Could you check a few things on this model? Use its own coordinates, in mm. Round coordinates to 2 decimals unless told otherwise and drop trailing zeros. Write each loop counter-clockwise with the first axis right and the second up, starting at its lowest first coordinate (ties: lowest second). Pieces come first, ordered by that corner, then holes. Notation, with made-up numbers: (31, 63.5) -> (78, 63.5) arc R22 cw to (78, 72.5) -> close; hole circle Ø2 at (4, 1). An arc over 180 degrees is marked (long way). Answer in a Markdown table with one row per item.
Autodesk Inventor part; units mm, degrees
ref_plane "YZ Plane" through (0, 0, 0) normal (1, 0, 0) x (0, 1, 0)
ref_plane "XZ Plane" through (0, 0, 0) normal (0, 1, 0) x (-1, 0, 0)
ref_plane "XY Plane" through (0, 0, 0) normal (0, 0, 1) x (1, 0, 0)
sketch "Sketch1" plane through (0, 0, 0) normal (0, 1, 0) x (-1, 0, 0)
  line L0 (945.4953, -52.3895) -> (1058.1259, -52.3895)
  arc A0 (945.4953, 55.8486) -> (981.8106, 103.6105) centre (854.964, 162.3701) ccw
  arc A1 (1021.8106, 103.6105) -> (1058.1259, 55.8486) centre (1148.6572, 162.3701) ccw
  line L1 (967.8106, 44.6105) -> (967.8106, 29.6105)
  line L2 (967.8106, -8.3895) -> (967.8106, -23.3895)
  line L3 (967.8106, 44.6105) -> (964.8106, 44.6105)
  line L4 (964.8106, 44.6105) -> (964.8106, 29.6105)
  line L5 (964.8106, 29.6105) -> (967.8106, 29.6105)
  line L6 (967.8106, -23.3895) -> (964.8106, -23.3895)
  line L7 (964.8106, -23.3895) -> (964.8106, -8.3895)
  line L8 (964.8106, -8.3895) -> (967.8106, -8.3895)
  line L9 (1035.8106, 44.6105) -> (1035.8106, 29.6105)
  line L10 (1035.8106, -8.3895) -> (1035.8106, -23.3895)
  line L11 (1035.8106, 44.6105) -> (1038.8106, 44.6105)
  line L12 (1038.8106, 44.6105) -> (1038.8106, 29.6105)
  line L13 (1038.8106, 29.6105) -> (1035.8106, 29.6105)
  line L14 (1035.8106, -23.3895) -> (1038.8106, -23.3895)
  line L15 (1038.8106, -23.3895) -> (1038.8106, -8.3895)
  line L16 (1038.8106, -8.3895) -> (1035.8106, -8.3895)
  line L17 (1058.1259, 55.8486) -> (1058.1259, -52.3895)
  line L18 (945.4953, 55.8486) -> (945.4953, -52.3895)
  line L19 (1001.8106, 123.6105) -> (1003.3106, 123.6105)
  line L20 (1003.3106, 123.6105) -> (1003.3106, 115.6105)
  line L21 (1003.3106, 111.6105) -> (1000.3106, 111.6105)
  line L22 (1000.3106, 115.6105) -> (1000.3106, 123.6257)
  line L23 (1000.3106, 123.6257) -> (1001.8106, 123.6105)
  line L24 (1003.3106, 115.6105) -> (1003.3106, 111.6105)
  line L25 (1000.3106, 115.6105) -> (1000.3106, 111.6105)
  arc A2 (1012.3106, 159.6326) -> (991.3106, 159.6326) centre (1001.8106, 142.6105) ccw
  arc A3 (981.8106, 103.6105) -> (991.3106, 159.6326) centre (700.3575, 180.1548) ccw
  arc A4 (1012.3106, 159.6326) -> (1021.8106, 103.6105) centre (1303.2637, 180.1548) ccw
  arc A5 (945.4953, 55.8486) -> (981.8106, 103.6105) centre (854.964, 162.3701) ccw
  arc A6 (1021.8106, 103.6105) -> (1058.1259, 55.8486) centre (1148.6572, 162.3701) ccw
  line L26 (1001.8106, 123.6105) -> (1003.3106, 123.6105)
  line L27 (1003.3106, 123.6105) -> (1003.3106, 115.6105)
  line L28 (1003.3106, 111.6105) -> (1000.3106, 111.6105)
  line L29 (1000.3106, 115.6105) -> (1000.3106, 123.6105)
  line L30 (1000.3106, 123.6105) -> (1001.8106, 123.6105)
  line L31 (1000.3106, 111.6105) -> (1000.3106, 115.6105)
  line L32 (1003.3106, 111.6105) -> (1003.3106, 115.6105)
  line L33 (1001.8106, 103.6105) -> (1086.8106, 103.6105) construction
  line L34 (1001.8106, 103.6105) -> (916.8106, 103.6105) construction
  line L35 (1086.8106, 133.6105) -> (1071.8106, 133.6105) construction
  line L36 (1071.8106, 133.6105) -> (1071.8106, 73.6105) construction
  line L37 (1071.8106, 73.6105) -> (1101.8106, 73.6105) construction
  line L38 (1101.8106, 73.6105) -> (1101.8106, 133.6105) construction
  line L39 (1101.8106, 133.6105) -> (1086.8106, 133.6105) construction
  line L40 (916.8106, 133.6105) -> (931.8106, 133.6105) construction
  line L41 (931.8106, 133.6105) -> (931.8106, 73.6105) construction
  line L42 (931.8106, 73.6105) -> (901.8106, 73.6105) construction
  line L43 (901.8106, 73.6105) -> (901.8106, 133.6105) construction
  line L44 (901.8106, 133.6105) -> (916.8106, 133.6105) construction
  line L45 (931.8106, 103.6105) -> (935.8106, 103.6105) construction
  line L46 (935.8106, 103.6105) -> (935.8106, 108.6105) construction
  line L47 (1071.8106, 103.6105) -> (1067.8106, 103.6105) construction
  line L48 (1067.8106, 103.6105) -> (1067.8106, 108.6105) construction
  line L49 (935.8106, 103.6105) -> (939.8106, 103.6105) construction
  line L50 (1067.8106, 103.6105) -> (1063.8106, 103.6105) construction
  line L51 (939.8106, 103.6105) -> (949.8106, 103.6105) construction
  line L52 (949.8106, 103.6105) -> (996.7952, 86.5095) construction
  line L53 (949.8106, 103.6105) -> (996.7952, 120.7115) construction
  line L54 (1063.8106, 103.6105) -> (1053.8106, 103.6105) construction
  line L55 (1053.8106, 103.6105) -> (1006.826, 120.7115) construction
  line L56 (1053.8106, 103.6105) -> (1006.826, 86.5095) construction
  line L57 (939.8106, 103.6105) -> (952.4597, 65.6632) construction
  line L58 (952.4597, 65.6632) -> (1051.1615, 65.6632) construction
  line L59 (1051.1615, 65.6632) -> (1063.8106, 103.6105) construction
  line L60 (1001.8106, 123.6105) -> (1001.8106, 168.6105) construction
  line L61 (1001.8106, 123.6105) -> (1003.3106, 123.6105)
  line L62 (1003.3106, 123.6105) -> (1003.3106, 115.6105)
  line L63 (1003.3106, 111.6105) -> (1000.3106, 111.6105)
  line L64 (1000.3106, 115.6105) -> (1000.3106, 123.6257)
  line L65 (1000.3106, 123.6257) -> (1001.8106, 123.6105)
  line L66 (1003.3106, 115.6105) -> (1003.3106, 111.6105)
  line L67 (1000.3106, 115.6105) -> (1000.3106, 111.6105)
  arc A7 (1012.3106, 159.6326) -> (991.3106, 159.6326) centre (1001.8106, 142.6105) ccw
  arc A8 (981.8106, 103.6105) -> (991.3106, 159.6326) centre (700.3575, 180.1548) ccw
  arc A9 (1012.3106, 159.6326) -> (1021.8106, 103.6105) centre (1303.2637, 180.1548) ccw
  line L68 (1001.8106, 78.6105) -> (1006.8106, 78.6105) construction
  line L69 (1006.8106, 78.6105) -> (1006.8106, 128.6105) construction
  line L70 (1006.8106, 128.6105) -> (996.8106, 128.6105) construction
  line L71 (996.8106, 128.6105) -> (996.8106, 78.6105) construction
  line L72 (996.8106, 78.6105) -> (1001.8106, 78.6105) construction
  circle A10 centre (1006.8106, 78.6105) radius 2.25
  circle A11 centre (996.8106, 78.6105) radius 2.25
  circle A12 centre (1006.8106, 128.6105) radius 2.25
  circle A13 centre (996.8106, 128.6105) radius 2.25
  point P0 (0, 0)
extrude "Extrusion1" add sketch "Sketch1" along normal blind 3
ref_plane "Work Plane1" through (-1001.8106, 0, 55.8486) normal (1, 0, 0) x (0, 0, -1)
properties part number "上底盤新"
1) For pin 1 (0.9 mm diameter, centred on y = 1, z = 118.5, fed in from -X); pin 2 (1.5 mm diameter, centred on x = -1002.5, y = 1.5, fed in from +Z), each with a flat end and sliding along its axis, tell me the tip position at first contact or that it passes through.
Findings:
| item | result |
|---|---|
| pin 1 | stops at x = -1018.28 |
| pin 2 | stops at z = 162.61 |
2) Thinking about a two-plate mould opening in X: for faces 1 (the face through (-1008.957, 1.479, 127.935)), 2 (the face through (-1015.76, 1.48, 131)), 3 (the face through (-987.994, 1.479, 131.782)), 4 (the face through (-1001, 0, 33)), which applies, +X half, -X half, draft (parallel to the pull), parting line (faces both ways), or undercut?
Findings:
| item | result |
|---|---|
| face 1 | undercut |
| face 2 | -X half |
| face 3 | +X half |
| face 4 | draft |
3) Please list where these lines run through material, in increasing order: line 1 (X direction, y = 0.65, z = 39.5); line 2 (Z direction, x = -995, y = 1.4); line 3 (Z direction, x = -966, y = 2.7).
Findings:
| item | result |
|---|---|
| line 1 | x = -1058.13 to -1038.81, -1035.81 to -967.81, -964.81 to -945.5 |
| line 2 | z = -52.39 to 77.27, 79.95 to 127.27, 129.95 to 161.42 |
| line 3 | z = -52.39 to -23.39, -8.39 to 29.61, 44.61 to 77.44 |
4) Imagine slicing it at A-A, the plane y = 2.4. Count the separate pieces of the cut face and the enclosed holes in it, plus the area to 3 significant figures.
Findings:
| item | result |
|---|---|
| separate pieces | 1 |
| enclosed holes | 9 |
| area | 16,900 mm^2 |
5) Imagine slicing it at C-C, the plane z = 139.5. Please give me the cut outline in (x, y), plus the area to 3 significant figures.
Findings:
| item | result |
|---|---|
| outline | (-1014.43, 0) -> (-989.19, 0) -> (-989.19, 3) -> (-1014.43, 3) -> close |
| area | 75.7 mm^2 |
6) Imagine slicing it at B-B, the plane x = -1025. Please give me the cut outline in (y, z), plus the area to 3 significant figures.
Findings:
| item | result |
|---|---|
| outline | (0, -52.39) -> (3, -52.39) -> (3, 97.17) -> (0, 97.17) -> close |
| area | 449 mm^2 |
